from build123d import *

# Parameters (mm, degrees)
SKETCH1_R           = 1.075
SKETCH1_R_2         = 1.375
BOSS_EXTRUDE1_DEPTH = 3
BOSS_EXTRUDE2_DEPTH = 4
SKETCH3_R           = 1.575
CUT_EXTRUDE1_DEPTH  = 10


with BuildPart() as part:
    # Sketch1 → Boss-Extrude1 (new body)
    with BuildSketch(Plane.XY):
        with BuildLine():
            Line((-26.25, 89.183481687), (-26.25, 39.183481687))
            ThreePointArc((-26.25, 39.183481687), (-16.25, 29.183481687), (-6.25, 39.183481687))
            Line((-6.25, 39.183481687), (-6.25, 79.183481687))
            ThreePointArc((-6.25, 79.183481687), (-9.178932188, 86.254549499), (-16.25, 89.183481687))
            Line((-16.25, 89.183481687), (-26.25, 89.183481687))
        make_face()
        with Locations((-16.298780591, 55.283407788)):
            Circle(SKETCH1_R, mode=Mode.SUBTRACT)
        with Locations((-16.25, 39.183481687)):
            Circle(SKETCH1_R_2, mode=Mode.SUBTRACT)
    extrude(amount=BOSS_EXTRUDE1_DEPTH)

    # Sketch1_4 → Boss-Extrude2 (add)
    with BuildSketch(Plane.XY):
        with BuildLine():
            Line((-19.535875527, 55.989457894), (-21.249709959, 39.23733634))
            ThreePointArc((-21.249709959, 39.23733634), (-16.248864162, 34.183481816), (-11.250315025, 39.239607879))
            Line((-11.250315025, 39.239607879), (-13.036870696, 55.991806015))
            ThreePointArc((-13.036870696, 55.991806015), (-16.287526809, 59.183775163), (-19.535875527, 55.989457894))
        make_face()
        with BuildLine():
            ThreePointArc((-14.036352569, 55.933775375), (-16.286352569, 58.183775375), (-18.536352569, 55.933775375))
            Line((-18.536352569, 55.933775375), (-20.25, 39.183481687))
            ThreePointArc((-20.25, 39.183481687), (-16.25, 35.183481687), (-12.25, 39.183481687))
            Line((-12.25, 39.183481687), (-14.036352569, 55.933775375))
        make_face(mode=Mode.SUBTRACT)
    extrude(amount=-BOSS_EXTRUDE2_DEPTH)

    # Sketch3 → Cut-Extrude1 (cut)
    with BuildSketch(Plane.XY.offset(3)):
        with Locations((-16.25, 79.183481687)):
            Circle(SKETCH3_R)
    extrude(amount=-CUT_EXTRUDE1_DEPTH, mode=Mode.SUBTRACT)


solid = part.part
Part model, mm, in its own coordinate system. A direction names the side the tool comes from. Coordinates: 2 decimals unless noted, no trailing zeros. Write each loop counter-clockwise with the first axis right and the second up, starting at its lowest first coordinate (ties: lowest second). Pieces come first, ordered by that corner, then holes. Notation, with made-up numbers: M -9.75,60.25 L 17.25,60.25 A26 ccw 17.25,90.25 Z; hole C 84.5,51 d9. An arc over 180 degrees is marked long. Return JSON: item names as keys, results as strings.
1. Flat gauge pin, fed straight in: pin 1 Ø1 at (x, y) = (-18.5, 49.5) entering from -Z. Where does the tip first touch, or does it go through?
Determined:
{"pin 1": "z = 0"}
2. Saw through at C-C, the plane y = 41.5. Write the cut outline in (x, z).
Determined:
{"outline": "M -26.25,0 L -21.02,0 L -21.02,-4 L -20.01,-4 L -20.01,0 L -12.5,0 L -12.5,-4 L -11.49,-4 L -11.49,0 L -6.25,0 L -6.25,3 L -26.25,3 Z"}
3. Saw through at A-A, the plane z = -2. Write the cut outline in (x, y).
Determined:
{"outline": "M -21.25,39.24 A5 ccw long -11.25,39.24 L -13.04,55.99 A3.25 ccw -19.54,55.99 Z; hole M -20.25,39.18 A4 ccw -12.25,39.18 L -14.04,55.93 A2.25 ccw -18.54,55.93 Z"}
4. Pull direction X, two halves, no side cores. Call faces 4 (the face through (-16.338, 35.184, -1.972)), 5 (the face through (-21, 89.183, 1)), 6 (the face through (-16.47, 29.186, 1.479)): pulls with the +X half, pulls with the -X half, needs draft (parallel to the pull), parting line crosses it, or undercut.
Determined:
{"face 4": "undercut", "face 5": "needs draft", "face 6": "parting line crosses it"}
5. Saw through at D-D, the plane x = -23.25. Write the cut outline in (y, z).
Determined:
{"outline": "M 32.04,0 L 89.18,0 L 89.18,3 L 32.04,3 Z"}
6. 3-axis set-ups, long thin cutter, end or side, ignore diameter. For faces 1 (the face through (-19.38, 47.68, -1.97)), 2 (the face through (-12.13, 47.5, -1.97)), 3 (the face through (-20.38, 47.73, -1.97)): which of +Z, -Z, +X, -X, +Y, -Y reach the whole face in a straight line?
Determined:
{"face 1": "-Z", "face 2": "-Z, +X, +Y", "face 3": "-Z, -X, +Y"}
7. Probe L1, parallel to Y at x = -16.25, z = 0.8; L2, parallel to Z at x = -17.75, y = 57.5; L3, parallel to X at y = 37, z = -1.5. List the from-to ranges inside material, lowest first.
Determined:
{"L1": "29.18 to 37.81, 40.56 to 54.21, 56.36 to 77.61, 80.76 to 89.18", "L2": "0 to 3", "L3": "-20.75 to -19.6, -12.9 to -11.75"}
8. Saw through at B-B, the plane z = 1.5. Write the cut outline in (x, y) (3 decimals), then the cut area to 3 significant figures.
Determined:
{"outline": "M -26.25,39.183 A10 ccw -6.25,39.183 L -6.25,79.183 A10 ccw -16.25,89.183 L -26.25,89.183 Z; hole C -16.25,79.183 d3.15; hole C -16.25,39.183 d2.75; hole C -16.299,55.283 d2.15", "area": "1,120 mm²"}
